Here's the drawing with two shaded views (mm, measured from the low corner). I have some questions. Coordinates: 2 decimals unless noted, no trailing zeros. Write each loop counter-clockwise with the first axis right and the second up, starting at its lowest first coordinate (ties: lowest second). Pieces come first, ordered by that corner, then holes. Notation, with made-up numbers: (-17, 36) -> (13, 36) arc R10 ccw to (13, 46) -> close; hole circle Ø6 at (-14, 51.25). An arc over 180 degrees is marked (long way). Use one line per item in the form item = value.
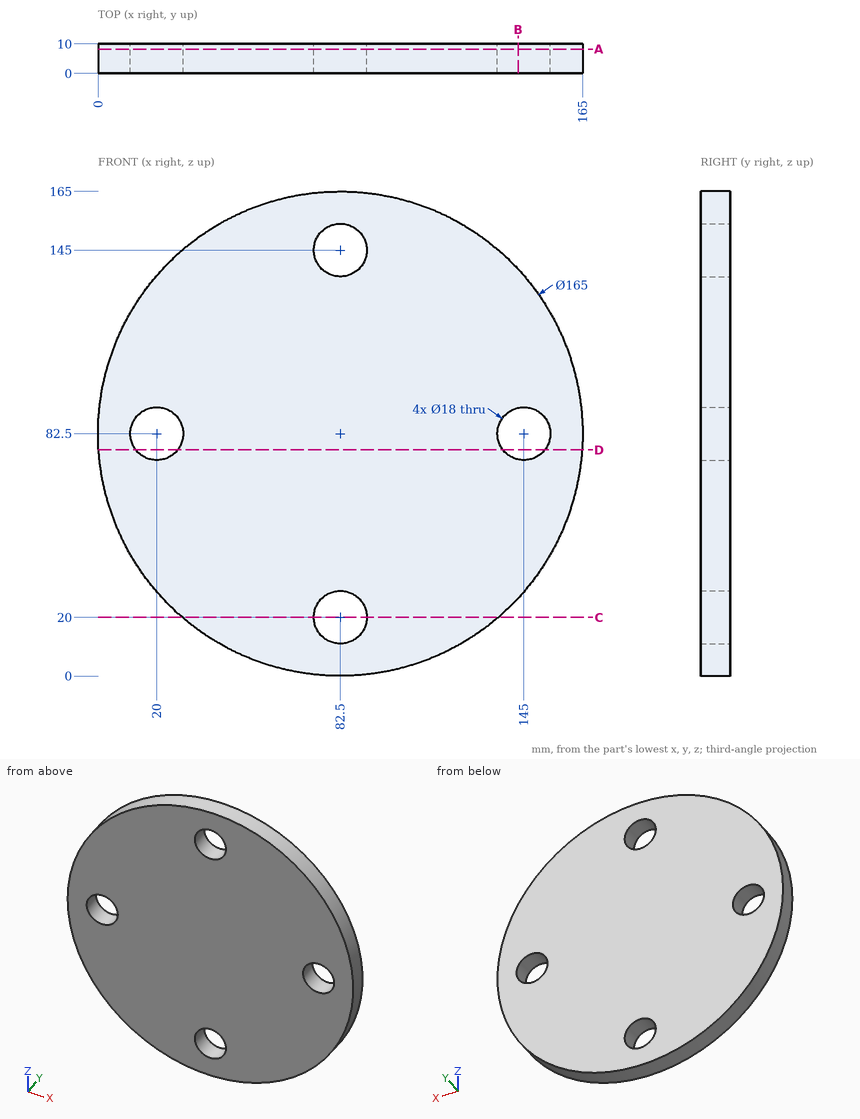
Q1. Suppose I cut it at B-B (x = 143). Write out the boundary of the cut face in (y, z).
Return value:
outline = (0, 26.41) -> (10, 26.41) -> (10, 73.73) -> (0, 73.73) -> close; (0, 91.27) -> (10, 91.27) -> (10, 138.59) -> (0, 138.59) -> close
Q2. Suppose I cut it at D-D (z = 77). Write out the boundary of the cut face in (x, y).
Return value:
outline = (0.18, 0) -> (12.88, 0) -> (12.88, 10) -> (0.18, 10) -> close; (27.12, 0) -> (137.88, 0) -> (137.88, 10) -> (27.12, 10) -> close; (152.12, 0) -> (164.82, 0) -> (164.82, 10) -> (152.12, 10) -> close
Q3. Suppose I cut it at A-A (y = 8.25). Write out the boundary of the cut face in (x, z).
Return value:
outline = circle Ø165 at (82.5, 82.5); hole circle Ø18 at (20, 82.5); hole circle Ø18 at (82.5, 20); hole circle Ø18 at (82.5, 145); hole circle Ø18 at (145, 82.5)
Q4. Suppose I cut it at C-C (z = 20). Write out the boundary of the cut face in (x, y), then the cut area to 3 significant figures.
Return value:
outline = (28.65, 0) -> (73.5, 0) -> (73.5, 10) -> (28.65, 10) -> close; (91.5, 0) -> (136.35, 0) -> (136.35, 10) -> (91.5, 10) -> close
area = 897 mm2
Q5. Will these pins go through, and if not, where does the flat tip stop? pin 1 (11 mm diameter, centred on x = 82.5, z = 145, fed in from +Y); pin 2 (5 mm diameter, centred on x = 102.5, y = 7.5, fed in from +Z); pin 3 (1.5 mm diameter, centred on x = 66.5, y = 8, fed in from -Z); pin 4 (2 mm diameter, centred on y = 7, z = 123, fed in from +X).
Return value:
pin_1 = through
pin_2 = 163.12
pin_3 = 1.42
pin_4 = 154.93
Q6. If I drill on line 1 (Z direction, x = 82.5, y = 3.5); line 2 (X direction, y = 3, z = 84); line 3 (X direction, y = 7, z = 145), over which ranges is the centre line in solid material (lowest first)? Write a range as from..to.
Return value:
line_1 = 0..11, 29..136, 154..165
line_2 = 0.01..11.13, 28.87..136.13, 153.87..164.99
line_3 = 28.65..73.5, 91.5..136.35
